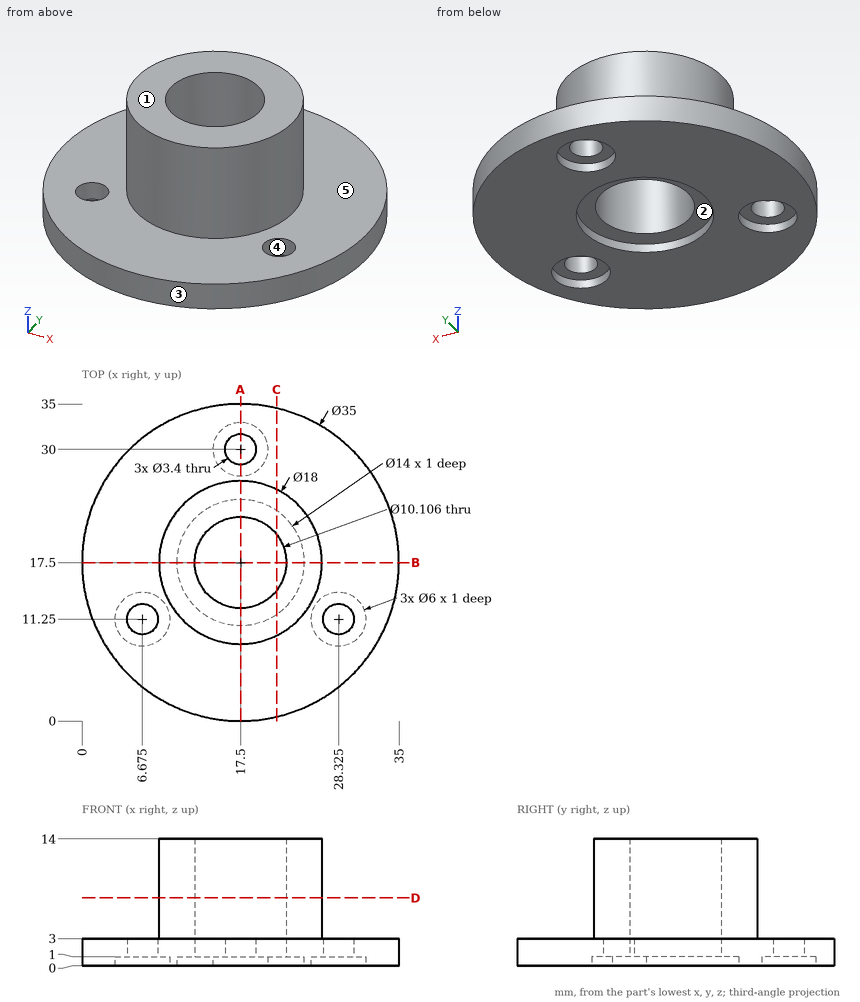
Can you work these out from the drawing? Everything is in mm from the part's minimum corner. A direction names the side the tool comes from. Round coordinates to 2 decimals unless told otherwise and drop trailing zeros. Order: outer loops, then holes, each group sorted by start corner. A loop starts at its lowest first (then second) coordinate and runs counter-clockwise, first axis right, second up. Notation, with made-up numbers: (-36, -4.5) -> (-30, -4.5) arc R28 ccw to (-30, 27.5) -> close; hole circle Ø6 at (53, 64). An arc over 180 degrees is marked (long way). Return JSON: item names as keys, results as strings. Group by question number.
1. We'd pull the mould along Y, two halves only. Please class the marked faces 1, 2 and 3: released by +Y, released by -Y, zero draft, split by the parting line, or undercut.
2. If we section it at C-C, the plane x = 21.5: Write out the boundary of the cut face in (y, z) (1 decimal), then the cut area to 3 significant figures.
3. If we section it at D-D, the plane z = 7.5: Write out the boundary of the cut face in (x, y).
4. Which directions (+Z, -Z, +X, -X, +Y, -Y) give clear straight access to the entire face, cutting with the end or side of a thin tool? Please do the marked faces 4 and 5.
5. If we section it at B-B, the plane y = 17.5: Write out the boundary of the cut face in (x, z), then the cut area to 3 significant figures.
6. I need wall thicknesses on line 1 (Y direction, x = 17.5, z = 0.35); line 2 (X direction, y = 11.25, z = 2.5) (1 decimal); line 3 (Y direction, x = 17.5, z = 10.75). Which ranges of each line are inside material? Lowest first, please. Write a range as [from, to].
7. If we section it at A-A, the plane x = 17.5: Write out the boundary of the cut face in (y, z), then the cut area to 3 significant figures.
8. Will these pins go through, and if not, where does the flat tip stop? pin 1 (4.5 mm diameter, centred on x = 17.5, y = 30, fed in from -Z); pin 2 (3 mm diameter, centred on y = 12, z = 5.5, fed in from +X); pin 3 (5.5 mm diameter, centred on x = 28.33, y = 11.25, fed in from +Z); pin 4 (4 mm diameter, centred on x = 15, y = 19, fed in from +Z).
Output values:
{
 "1": {"face 1": "zero draft", "face 2": "undercut", "face 3": "split by the parting line"},
 "2": {"outline": "(0.5, 0) -> (11.8, 0) -> (11.8, 1) -> (14.4, 1) -> (14.4, 14) -> (9.4, 14) -> (9.4, 3) -> (0.5, 3) -> close; (20.6, 1) -> (23.2, 1) -> (23.2, 0) -> (34.5, 0) -> (34.5, 3) -> (25.6, 3) -> (25.6, 14) -> (20.6, 14) -> close", "area": "188 mm²"},
 "3": {"outline": "circle Ø18 at (17.5, 17.5); hole circle Ø10.11 at (17.5, 17.5)"},
 "4": {"face 4": "+Z, -Z", "face 5": "+Z"},
 "5": {"outline": "(0, 0) -> (10.5, 0) -> (10.5, 1) -> (12.45, 1) -> (12.45, 14) -> (8.5, 14) -> (8.5, 3) -> (0, 3) -> close; (22.55, 1) -> (24.5, 1) -> (24.5, 0) -> (35, 0) -> (35, 3) -> (26.5, 3) -> (26.5, 14) -> (22.55, 14) -> close", "area": "158 mm²"},
 "6": {"line 1": "[0, 10.5], [24.5, 27], [33, 35]", "line 2": "[1.2, 5], [8.4, 26.6], [30, 33.8]", "line 3": "[8.5, 12.45], [22.55, 26.5]"},
 "7": {"outline": "(0, 0) -> (10.5, 0) -> (10.5, 1) -> (12.45, 1) -> (12.45, 14) -> (8.5, 14) -> (8.5, 3) -> (0, 3) -> close; (22.55, 1) -> (24.5, 1) -> (24.5, 0) -> (27, 0) -> (27, 1) -> (28.3, 1) -> (28.3, 3) -> (26.5, 3) -> (26.5, 14) -> (22.55, 14) -> close; (31.7, 1) -> (33, 1) -> (33, 0) -> (35, 0) -> (35, 3) -> (31.7, 3) -> close", "area": "145 mm²"},
 "8": {"pin 1": "z = 1", "pin 2": "x = 25.56", "pin 3": "z = 3", "pin 4": "through"}
}
